Here's how the part is built. I have some questions about the finished solid (model axes, mm). A direction names the side the tool comes from. Coordinates: 2 decimals unless noted, no trailing zeros. Write each loop counter-clockwise with the first axis right and the second up, starting at its lowest first coordinate (ties: lowest second). Pieces come first, ordered by that corner, then holes.
Item 1: I want a section at C-C (x = 4). Please give me the cut outline in (y, z), and give its area (3 significant figures).
Item 2: Please list where these lines run through material, in increasing order: line 1 (X direction, y = 22.5, z = 12.5); line 2 (Y direction, x = 22, z = 3).
Item 3: If we mould it in two halves opening along X, with no side actions, what happens to faces 1 (the face through (-20, 25, 13.8)), 2 (the face through (-19.793, -26.908, 0.913)), 3 (the face through (20, -12, 1))? For each: pulls with the +X half, pulls with the -X half, needs draft (parallel to the pull), parting line crosses it, or undercut.
Item 4: For faces 4 (the face through (-18.807, -15.782, 6.279)), 5 (the face through (19.793, 26.908, 0.887)), 6 (the face through (12.5, 0, 1)), which set-ups out of +Z, -Z, +X, -X, +Y, -Y let a thin tool reach every point of the face, with its end or its side?
Item 5: I'm going to push flat-ended pins straight in: P1, Ø0.9, axis at x = 0.5, z = 1, coming from the -Y side; P2, Ø2, axis at x = -17.5, y = 17.5, coming from the +Z side; P3, Ø1.5, axis at x = 12.5, z = 9, coming from the +Y side; P4, Ø1.4, axis at x = 1, z = 1, coming from the +Y side. Where does each tip first touch, or does it pass through?
Item 6: I want a section at B-B (z = 7). Please give me the cut outline in (x, y), and give its area (3 significant figures).
Item 7: I want a section at A-A (z = 12.75). Please give me the cut outline in (x, y).
Item 8: I want a section at D-D (y = -22). Please give me the cut outline in (x, z).
from build123d import *

# Parameters (mm, degrees)
F0_W      = 55
F0_H      = 55
F1_DEPTH  = 1.8
F2_R      = 3.5
F3_DEPTH  = 3
F4_R      = 2.9
F5_DEPTH  = 3
F6_R      = 4.5
F7_DEPTH  = 12
F8_R      = 3.2
F9_DEPTH  = 12
F10_R     = 4
F11_W     = 15
F11_H     = 15
F12_DEPTH = 20
F14_DEPTH = 25
F15_R     = 8
F16_R     = 5


with BuildPart() as f1:
    # F0 (on Top) → F1 (new body)
    with BuildSketch(Plane.XY):
        Rectangle(F0_W, F0_H)
    extrude(amount=F1_DEPTH)

    # F2 (on face) → F3 (join)
    with BuildSketch(Plane.XY.offset(1.8)):
        with Locations((-15.9099025767, 15.9099025767)):
            Circle(F2_R)
        with Locations((15.9099025767, 15.9099025767)):
            Circle(F2_R)
        with Locations((-15.9099025767, -15.9099025767)):
            Circle(F2_R)
        with Locations((15.9099025767, -15.9099025767)):
            Circle(F2_R)
    extrude(amount=F3_DEPTH)

    # F4 (on face) → F5 (join)
    with BuildSketch(Plane.XY.offset(4.8)):
        with Locations((-15.9099025767, 15.9099025767)):
            Circle(F4_R)
        with Locations((15.9099025767, 15.9099025767)):
            Circle(F4_R)
        with Locations((-15.9099025767, -15.9099025767)):
            Circle(F4_R)
        with Locations((15.9099025767, -15.9099025767)):
            Circle(F4_R)
    extrude(amount=F5_DEPTH)

    # F6 (on face) → F7 (join)
    with BuildSketch(Plane.XY.offset(1.8)):
        with Locations((-22.627416998, 22.627416998)):
            Circle(F6_R)
        with Locations((22.627416998, 22.627416998)):
            Circle(F6_R)
        with Locations((22.627416998, -22.627416998)):
            Circle(F6_R)
        with Locations((-22.627416998, -22.627416998)):
            Circle(F6_R)
    extrude(amount=F7_DEPTH)

    # F8 (on face) → F9 (cut)
    with BuildSketch(Plane.XY.offset(13.8)):
        with Locations((-22.627416998, -22.627416998)):
            Circle(F8_R)
        with Locations((22.627416998, -22.627416998)):
            Circle(F8_R)
        with Locations((-22.627416998, 22.627416998)):
            Circle(F8_R)
        with Locations((22.627416998, 22.627416998)):
            Circle(F8_R)
    extrude(amount=-F9_DEPTH, mode=Mode.SUBTRACT)

    # F10
    f10_edges = [f1.edges().sort_by_distance(p)[0] for p in [
        (27.5, -27.5, 0.9),
        (-27.5, -27.5, 0.9),
        (-27.5, 27.5, 0.9),
        (27.5, 27.5, 0.9),
    ]]
    fillet(f10_edges, radius=F10_R)

    # F11 (on face) → F12 (cut, symmetric)
    with BuildSketch(Plane.XY.offset(1.8)):
        Polygon((-12.5, 4.5), (-27.5, 19.5), (-27.5, -19.5), (-12.5, -4.5), align=None)
        Polygon((19.5, 27.5), (-19.5, 27.5), (-4.5, 12.5), (4.5, 12.5), align=None)
        Polygon((27.5, -19.5), (27.5, 19.5), (12.5, 4.5), (12.5, -4.5), align=None)
        Polygon((-4.5, -12.5), (-19.5, -27.5), (19.5, -27.5), (4.5, -12.5), align=None)
        Rectangle(F11_W, F11_H)
    extrude(amount=F12_DEPTH, both=True, mode=Mode.SUBTRACT)

    # F13 (on face) → F14 (cut)
    with BuildSketch(Plane.XY.offset(1.8)):
        Polygon((-26.8456843913, 19.823363167), (-25.4314708289, 18.4091496047), (-22.6030437041, 21.2375767294), (-24.0172572665, 22.6517902918), align=None)
        Polygon((22.6030437041, 21.2375767294), (25.4314708289, 18.4091496047), (26.8456843913, 19.823363167), (24.0172572665, 22.6517902918), align=None)
        Polygon((-25.4314708289, -18.4091496047), (-26.8456843913, -19.823363167), (-24.0172572665, -22.6517902918), (-22.6030437041, -21.2375767294), align=None)
        Polygon((26.8456843913, -19.823363167), (25.4314708289, -18.4091496047), (22.6030437041, -21.2375767294), (24.0172572665, -22.6517902918), align=None)
    extrude(amount=F14_DEPTH, mode=Mode.SUBTRACT)

    # F15
    f15_edges = [f1.edges().sort_by_distance(p)[0] for p in [
        (19.5, -27.5, 0.9),
        (4.5, -12.5, 0.9),
        (-4.5, -12.5, 0.9),
        (-19.5, -27.5, 0.9),
        (-27.5, -19.5, 0.9),
        (-12.5, -4.5, 0.9),
        (-12.5, 4.5, 0.9),
        (-27.5, 19.5, 0.9),
        (-19.5, 27.5, 0.9),
        (-4.5, 12.5, 0.9),
        (4.5, 12.5, 0.9),
        (19.5, 27.5, 0.9),
        (12.5, -4.5, 0.9),
        (12.5, 4.5, 0.9),
        (27.5, 19.5, 0.9),
        (27.5, -19.5, 0.9),
    ]]
    fillet(f15_edges, radius=F15_R)

    # F16
    f16_edges = [f1.edges().sort_by_distance(p)[0] for p in [
        (-7.5, 7.5, 0.9),
        (7.5, 7.5, 0.9),
        (7.5, -7.5, 0.9),
        (-7.5, -7.5, 0.9),
    ]]
    fillet(f16_edges, radius=F16_R)


solid = f1.part
Answer:
1. outline: (-13.01, 0) - (-7.27, 0) - (-7.27, 1.8) - (-13.01, 1.8) - close; (7.27, 0) - (13.01, 0) - (13.01, 1.8) - (7.27, 1.8) - close
1. area: 20.7 mm2
2. line 1: x = -27.13 to -25.82, -19.43 to -18.13, 18.13 to 19.43, 25.82 to 27.13
2. line 2: y = -27.08 to -25.77, -19.49 to -18.17, 18.17 to 19.49, 25.77 to 27.08
3. face 1: needs draft
3. face 2: undercut
3. face 3: pulls with the +X half
4. face 4: +Z
4. face 5: +Z, -Z, +Y
4. face 6: +Z, -Z, +X
5. P1: stops at y = -12.5
5. P2: stops at z = 7.8
5. P3: passes through
5. P4: stops at y = 12.52
6. outline: (-26.44, -20.23) arc R4.5 ccw (long way) to (-25.02, -18.82) - (-24.07, -19.77) arc R3.2 cw (long way) to (-25.48, -21.19) - close; (-26.44, 20.23) - (-25.48, 21.19) arc R3.2 cw (long way) to (-24.07, 19.77) - (-25.02, 18.82) arc R4.5 ccw (long way) to start; circle Ø5.8 at (-15.91, -15.91); circle Ø5.8 at (-15.91, 15.91); circle Ø5.8 at (15.91, -15.91); circle Ø5.8 at (15.91, 15.91); (24.07, -19.77) - (25.02, -18.82) arc R4.5 ccw (long way) to (26.44, -20.23) - (25.48, -21.19) arc R3.2 cw (long way) to start; (24.07, 19.77) arc R3.2 cw (long way) to (25.48, 21.19) - (26.44, 20.23) arc R4.5 ccw (long way) to (25.02, 18.82) - close
6. area: 221 mm2
7. outline: (-26.44, -20.23) arc R4.5 ccw (long way) to (-25.02, -18.82) - (-24.07, -19.77) arc R3.2 cw (long way) to (-25.48, -21.19) - close; (-26.44, 20.23) - (-25.48, 21.19) arc R3.2 cw (long way) to (-24.07, 19.77) - (-25.02, 18.82) arc R4.5 ccw (long way) to start; (24.07, -19.77) - (25.02, -18.82) arc R4.5 ccw (long way) to (26.44, -20.23) - (25.48, -21.19) arc R3.2 cw (long way) to start; (24.07, 19.77) arc R3.2 cw (long way) to (25.48, 21.19) - (26.44, 20.23) arc R4.5 ccw (long way) to (25.02, 18.82) - close
8. outline: (-27.46, 0) - (-14, 0) - (-14, 1.8) - (-18.17, 1.8) - (-18.17, 13.8) - (-19.49, 13.8) - (-19.49, 1.8) - (-25.77, 1.8) - (-25.77, 13.8) - (-27.08, 13.8) - (-27.08, 1.8) - (-27.46, 1.8) - close; (14, 0) - (27.46, 0) - (27.46, 1.8) - (27.08, 1.8) - (27.08, 13.8) - (25.77, 13.8) - (25.77, 1.8) - (19.49, 1.8) - (19.49, 13.8) - (18.17, 13.8) - (18.17, 1.8) - (14, 1.8) - close
